from build123d import *

# Parameters (mm, degrees)
SKETCH_1_R          = 1.35
EXTRUDE_1_DEPTH     = 40
SKETCH_2_R          = 1
CUT_EXTRUDE_1_DEPTH = 40


with BuildPart() as part:
    # 草图1 → 凸台-拉伸1 (new body)
    with BuildSketch(Plane.XY):
        with BuildLine():
            Line((0, 0), (5.773502692, 10))
            Line((5.773502692, 10), (-7.5, 10))
            Line((-7.5, 10), (-7.5, -10))
            Line((-7.5, -10), (-5.773502692, -10))
            Line((-5.773502692, -10), (-5.357205868, -9.278952749))
            ThreePointArc((-5.357205868, -9.278952749), (-6.499558695, -7.254218423), (-4.174910918, -7.231157828))
            Line((-4.174910918, -7.231157828), (0, 0))
        make_face()
        with Locations((-5.3304244, 7.070781577)):
            Circle(SKETCH_1_R, mode=Mode.SUBTRACT)
    extrude(amount=EXTRUDE_1_DEPTH)

    # 草图2 → 切除-拉伸1 (cut)
    with BuildSketch(Plane(origin=(0, 0, 0), x_dir=(0, 0, -1), z_dir=(0.8660254037844399, -0.4999999999999977, 0))):
        with Locations(Location((-1.25, -4, 0), (0, 0, 90))):
            Circle(SKETCH_2_R)
        with Locations(Location((-38.75, -4, 0), (0, 0, 90))):
            Circle(SKETCH_2_R)
    extrude(amount=-CUT_EXTRUDE_1_DEPTH, mode=Mode.SUBTRACT)


solid = part.part
Model file for the job. Use its own axes, mm. Give positions to 0.01 mm unless a question says otherwise; leave off trailing zeros. Write each loop counter-clockwise with the first axis right and the second up, starting at its lowest first coordinate (ties: lowest second). Pieces come first, ordered by that corner, then holes. Notation, with made-up numbers: (-29.5, -19.75) - (-7.5, -19.75) arc R4 cw to (-7.5, -14.75) - close; hole circle Ø5 at (-12, 35.25). An arc over 180 degrees is marked (long way). Answer as CSV lines item,"result".
1. Drill centre lines: L1, parallel to Y at x = -6.5, z = 27; L2, parallel to Z at x = -4, y = -3.25; L3, parallel to Y at x = 0.5, z = 15. Where is each one in solid material? Low to high. Write a range as [from, to].
Responses:
L1,"y = [-10, -8.6], [-7.25, 6.4], [7.75, 10]"
L2,"z = [0, 0.67], [1.83, 38.17], [39.33, 40]"
L3,"y = [0.87, 10]"
2. Pin check, flat tips, straight feed: pin 1 (1 mm diameter, centred on x = 0.5, z = 33.5, fed in from -Y); pin 2 (4 mm diameter, centred on y = -1.5, z = 6.5, fed in from +X); pin 3 (3 mm diameter, centred on x = 3.5, z = 22.5, fed in from -Y). Stop position of each tip, or through.
Responses:
pin 1,"stops at y = 0"
pin 2,"stops at x = 0.29"
pin 3,"stops at y = 3.46"
3. Band-saw the part on C-C (y = -5.25). Write the cut outline in (x, z), and give its area (3 significant figures).
Responses:
outline,"(-7.5, 0) - (-3.03, 0) - (-3.03, 40) - (-7.5, 40) - close"
area,"179 mm2"
4. Band-saw the part on A-A (z = 5). Write the cut outline in (x, y).
Responses:
outline,"(-7.5, -10) - (-5.77, -10) - (-5.36, -9.28) arc R1.35 cw (long way) to (-4.17, -7.23) - (5.77, 10) - (-7.5, 10) - close; hole circle Ø2.7 at (-5.33, 7.07)"
5. Band-saw the part on B-B (x = 0.5). Write the cut outline in (y, z), and give its area (3 significant figures).
Responses:
outline,"(0.87, 0) - (10, 0) - (10, 40) - (0.87, 40) - close"
area,"365 mm2"
6. Two-plate mould, pull along X, no slides. Class faces 1 (the face through (-7.5, 0, 20)), 2 (the face through (-2, 2, 0)), 3 (the face through (-4.496, -0.956, 0.867)): +X half, -X half, draft (parallel to the pull), parting line (faces both ways), or undercut.
Responses:
face 1,"-X half"
face 2,"draft"
face 3,"undercut"
